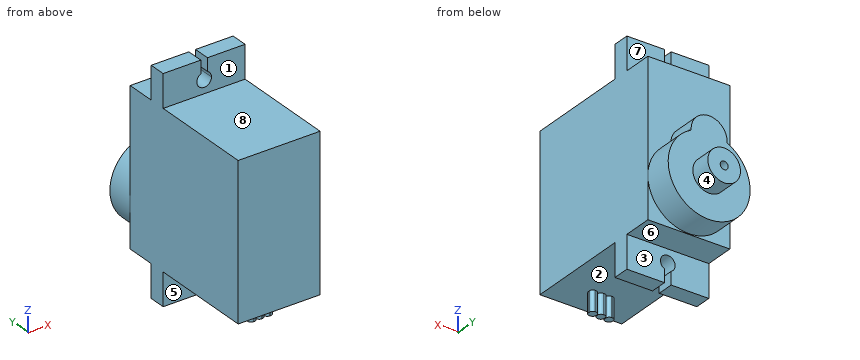
```python
from build123d import *

# Parameters (mm, degrees)
IZIM1_W                     = 12.3
IZIM1_H                     = 23
Y_KSEKLIK_EKSTR_ZYON1_DEPTH = 22.6
Y_KSEKLIK_EKSTR_ZYON2_DEPTH = 2.5
IZIM3_W                     = 3.6
IZIM3_H                     = 3
Y_KSEKLIK_EKSTR_ZYON3_DEPTH = 1.2
IZIM4_R                     = 6.15
Y_KSEKLIK_EKSTR_ZYON4_DEPTH = 4.25
IZIM5_R                     = 2.45
IZIM5_R_2                   = 0.6
Y_KSEKLIK_EKSTR_ZYON6_DEPTH = 3.15
IZIM6_W                     = 0.1
IZIM6_H                     = 1.2
KES_EKSTR_ZYON1_DEPTH       = 3
RADYUS1_R                   = 0.5


with BuildPart() as part:
    # Çizim1 → Yükseklik-Ekstrüzyon1 (new body)
    with BuildSketch(Plane(origin=(0, 0, 0), x_dir=(1, 0, 0), z_dir=(0, 1, 0))):
        Rectangle(IZIM1_W, IZIM1_H)
    extrude(amount=Y_KSEKLIK_EKSTR_ZYON1_DEPTH)

    # Çizim2 → Yükseklik-Ekstrüzyon2 (add)
    with BuildSketch(Plane(origin=(0, 18.2, 0), x_dir=(1, 0, 0), z_dir=(0, 1, 0))):
        with BuildLine():
            Line((-6.15, 16.4), (-6.15, -16.4))
            Line((-6.15, -16.4), (-0.5, -16.4))
            Line((-0.5, -16.4), (-0.5, -14.479795897))
            ThreePointArc((-0.5, -14.479795897), (-0.574456265, -12.561916848), (1.1, -13.5))
            ThreePointArc((1.1, -13.5), (0.938083152, -14.074456265), (0.5, -14.479795897))
            Line((0.5, -14.479795897), (0.5, -16.4))
            Line((0.5, -16.4), (6.15, -16.4))
            Line((6.15, -16.4), (6.15, 16.4))
            Line((6.15, 16.4), (0.5, 16.4))
            Line((0.5, 16.4), (0.5, 14.479795897))
            ThreePointArc((0.5, 14.479795897), (0.938083152, 14.074456265), (1.1, 13.5))
            ThreePointArc((1.1, 13.5), (-0.574456265, 12.561916848), (-0.5, 14.479795897))
            Line((-0.5, 14.479795897), (-0.5, 16.4))
            Line((-0.5, 16.4), (-6.15, 16.4))
        make_face()
    extrude(amount=-Y_KSEKLIK_EKSTR_ZYON2_DEPTH)

    # Çizim3 → Yükseklik-Ekstrüzyon3 (add)
    with BuildSketch(Plane(origin=(0, 4.8, 0), x_dir=(-1, 0, 0), z_dir=(0, -1, 0))):
        with Locations((0, 13)):
            Rectangle(IZIM3_W, IZIM3_H)
    extrude(amount=Y_KSEKLIK_EKSTR_ZYON3_DEPTH)

    # Çizim4 → Yükseklik-Ekstrüzyon4 (add)
    with BuildSketch(Plane(origin=(0, 22.6, 0), x_dir=(1, 0, 0), z_dir=(0, 1, 0))):
        with Locations((0, 5.25)):
            Circle(IZIM4_R)
        with BuildLine():
            Line((-2.7, -0.275622137), (-2.7, -0.5))
            ThreePointArc((-2.7, -0.5), (0, -3.2), (2.7, -0.5))
            Line((2.7, -0.5), (2.7, -0.275622137))
            ThreePointArc((2.7, -0.275622137), (0, -0.9), (-2.7, -0.275622137))
        make_face()
    extrude(amount=Y_KSEKLIK_EKSTR_ZYON4_DEPTH)

    # Çizim5 → Yükseklik-Ekstrüzyon6 (add)
    with BuildSketch(Plane(origin=(0, 26.85, 0), x_dir=(1, 0, 0), z_dir=(0, 1, 0))):
        with Locations(Location((0, 5.25, 0), (0, 0, 90))):
            Circle(IZIM5_R)
        with Locations(Location((0, 5.25, 0), (0, 0, 270))):
            Circle(IZIM5_R_2, mode=Mode.SUBTRACT)
    extrude(amount=Y_KSEKLIK_EKSTR_ZYON6_DEPTH)

    # Çizim6 → Kes-Ekstrüzyon1 (cut)
    with BuildSketch(Plane(origin=(0, 0, -14.5), x_dir=(-1, 0, 0), z_dir=(0, 0, -1))):
        with Locations((-0.616666667, 4.2)):
            Rectangle(IZIM6_W, IZIM6_H)
        with Locations((0.616666667, 4.2)):
            Rectangle(IZIM6_W, IZIM6_H)
    extrude(amount=-KES_EKSTR_ZYON1_DEPTH, mode=Mode.SUBTRACT)

    # Radyus1
    radyus1_edges = [part.edges().sort_by_distance(p)[0] for p in [
        (0.566666667, 3.6, -13),
        (0.566666667, 4.8, -13),
        (0.666666667, 4.8, -13),
        (0.666666667, 3.6, -13),
        (-0.666666667, 3.6, -13),
        (-0.666666667, 4.8, -13),
        (-0.566666667, 4.8, -13),
        (-0.566666667, 3.6, -13),
        (1.8, 4.8, -13),
        (-1.8, 4.8, -13),
        (1.8, 3.6, -13),
        (-1.8, 3.6, -13),
    ]]
    fillet(radyus1_edges, radius=RADYUS1_R)


solid = part.part
```
Can you work these out from the model? Positions are in its coordinate system, mm. Face numbers are marked on the shaded views. A direction names the side the tool comes from. Round coordinates to 2 decimals unless told otherwise and drop trailing zeros. Loops run counter-clockwise (first coordinate to the right, second up) from the corner with the lowest first, then second, coordinate; pieces in that order, holes last. Notation, with made-up numbers: (29, 50.5) -> (47, 50.5) arc R21 cw to (47, 60.5) -> close; hole circle Ø1 at (-28, 78). An arc over 180 degrees is marked (long way). Answer in a Markdown table with one row per item.
Item 1: Suppose I cut it at D-D, the plane z = -9. List the corners of the cut face in (x, y) for me.
Answer block:
| item | result |
|---|---|
| outline | (-6.15, 0) -> (6.15, 0) -> (6.15, 22.6) -> (4.87, 22.6) -> (4.87, 26.85) -> (-4.87, 26.85) -> (-4.87, 22.6) -> (-6.15, 22.6) -> close |
Item 2: Will these pins go through, and if not, where does the flat tip stop? P1, Ø1.2, axis at x = -1.5, y = 4.5, coming from the -Z side; P2, Ø1.5, axis at x = 1, y = 5, coming from the +Z side; P3, Ø6, axis at x = -1, y = 8, coming from the -Z side.
Answer block:
| item | result |
|---|---|
| P1 | z = -14.5 |
| P2 | z = 11.5 |
| P3 | z = -11.5 |
Item 3: We'd pull the mould along Y, two halves only. Please class the marked faces 1, 2 and 3: released by +Y, released by -Y, zero draft, split by the parting line, or undercut.
Answer block:
| item | result |
|---|---|
| face 1 | released by -Y |
| face 2 | undercut |
| face 3 | released by +Y |
Item 4: If I drill on probe 1 along X at (y, z) = (17.35, -13.5); probe 2 along Y at (x, z) = (-3, 9); probe 3 along X at (y, z) = (28.95, -5.25), over which ranges is the centre line in solid material (lowest first)?
Answer block:
| item | result |
|---|---|
| probe 1 | -6.15 to -1.1, 1.1 to 6.15 |
| probe 2 | 0 to 22.6 |
| probe 3 | -2.45 to -0.6, 0.6 to 2.45 |
Item 5: Suppose I cut it at C-C, the plane x = 4.75. List the corners of the cut face in (y, z) for me, plus the area to 3 significant figures.
Answer block:
| item | result |
|---|---|
| outline | (0, -11.5) -> (15.7, -11.5) -> (15.7, -16.4) -> (18.2, -16.4) -> (18.2, -11.5) -> (22.6, -11.5) -> (22.6, -9.16) -> (26.85, -9.16) -> (26.85, -1.34) -> (22.6, -1.34) -> (22.6, 11.5) -> (18.2, 11.5) -> (18.2, 16.4) -> (15.7, 16.4) -> (15.7, 11.5) -> (0, 11.5) -> close |
| area | 578 mm² |
Item 6: Suppose I cut it at A-A, the plane y = 16.25. List the corners of the cut face in (x, z) for me, plus the area to 3 significant figures.
Answer block:
| item | result |
|---|---|
| outline | (-6.15, -16.4) -> (-0.5, -16.4) -> (-0.5, -14.48) arc R1.1 cw (long way) to (0.5, -14.48) -> (0.5, -16.4) -> (6.15, -16.4) -> (6.15, 16.4) -> (0.5, 16.4) -> (0.5, 14.48) arc R1.1 cw (long way) to (-0.5, 14.48) -> (-0.5, 16.4) -> (-6.15, 16.4) -> close |
| area | 392 mm² |
Item 7: Suppose I cut it at B-B, the plane z = 7. List the corners of the cut face in (x, y) for me, plus the area to 3 significant figures.
Answer block:
| item | result |
|---|---|
| outline | (-6.15, 0) -> (6.15, 0) -> (6.15, 22.6) -> (-6.15, 22.6) -> close |
| area | 278 mm² |
Item 8: On a 3-axis mill with a long thin cutter (end or side, diameter ignored), from which of +Z, -Z, +X, -X, +Y, -Y can I reach the whole of each face in a straight line? I mean the marked faces 4, 5, 6, 7 and 8. Say none if no direction works.
Answer block:
| item | result |
|---|---|
| face 4 | +Y |
| face 5 | -Z, +X, -X |
| face 6 | -Z, +X, -X, +Y |
| face 7 | +Z, +X, -X, +Y |
| face 8 | +Z, +X, -X, -Y |
